Here's how the part is built. I have some questions about the finished solid (model axes, mm). Coordinates: 2 decimals unless noted, no trailing zeros. Loops run counter-clockwise (first coordinate to the right, second up) from the corner with the lowest first, then second, coordinate; pieces in that order, holes last. Notation, with made-up numbers: M 88,27 L 109,27 A31 ccw 109,62 Z; hole C 54,23.25 d5. An arc over 180 degrees is marked long. Use CSV: the item, a comma, the result in double quotes. Start each with the question number.
Q1. If we section it at D-D (y = 5): State how many separate pieces and enclosed holes the cut face has, and give its area (3 significant figures).
Q2. Please list where these lines run through material, in increasing order: probe 1 along X at (y, z) = (5, -1.55); probe 2 along Y at (x, z) = (-45, -2.2); probe 3 along Y at (x, z) = (-65, 0). Write a range as [from, to].
Q3. If we mould it in two halves opening along Y, with no side actions, what happens to faces 1 (the flat face through (-1, 0, 5)), 2 (the conical face through (-22.059, 3.125, 2.188)), 3 (the flat face through (1, 25, 0)), 4 (the cylindrical face through (-22.07, 3.48, -1.55))? For each: +Y half, -Y half, draft (parallel to the pull), parting line (faces both ways), or undercut.
Q4. For pin 1 Ø6 at (x, y) = (-25, 5) entering from -Z, with a flat end and sliding along its axis, tell me the tip position at first contact or that it passes through.
Q5. If we section it at B-B (z = -2): Please give me the cut outline in (x, y).
Q6. If we section it at A-A (x = -25): Please give me the cut outline in (y, z).
Q7. If we section it at C-C (x = -45): Please give me the cut outline in (y, z), and give its area (3 significant figures).
Autodesk Inventor part; units mm, degrees
ref_plane "YZ Plane" through (0, 0, 0) normal (1, 0, 0) x (0, 1, 0)
ref_plane "XZ Plane" through (0, 0, 0) normal (0, 1, 0) x (-1, 0, 0)
ref_plane "XY Plane" through (0, 0, 0) normal (0, 0, 1) x (1, 0, 0)
sketch "Sketch2" plane through (0, 0, 0) normal (0, 0, 1) x (1, 0, 0)
  line L0 (-75, -25) -> (75, -25)
  line L1 (75, -25) -> (75, 25)
  line L2 (75, 25) -> (-75, 25)
  line L3 (-75, 25) -> (-75, -25)
  line L4 (-75, -25) -> (75, 25) construction
  line L5 (75, -25) -> (-75, 25) construction
  point P0 (0, 0)
  dimension "d1" = 150
  dimension "d2" = 50
extrude "Extrusion1" add sketch "Sketch2" along normal mid plane 10
sketch "Sketch3" plane through (0, 0, 5) normal (0, 0, 1) x (1, 0, 0)
  line L0 (-75, 25) -> (-75, -25)
  line L1 (75, 25) -> (-75, 25)
  point P0 (0, 0)
  point P1 (-65, 0)
  dimension "d40" = 10
  dimension "d43" = 25
hole "Hole1" at (-65, 0, 5) direction (0, 0, -1) diameter 6.6 depth 14.2 tip angle 118 countersink diameter 12.6 countersink angle 90
sketch "Sketch4" plane through (0, 0, 5) normal (0, 0, 1) x (1, 0, 0)
  line L0 (-75, 25) -> (-75, -25)
  line L1 (75, 25) -> (-75, 25)
  point P0 (0, 0)
  point P1 (-45, 5)
  dimension "d41" = 30
  dimension "d42" = 20
hole "Hole2" at (-45, 5, 5) direction (0, 0, -1) diameter 9 depth 14.2 tip angle 118 countersink diameter 17.3 countersink angle 90
sketch "Sketch5" plane through (0, 0, 5) normal (0, 0, 1) x (1, 0, 0)
  line L0 (-75, 25) -> (-75, -25)
  line L1 (75, 25) -> (-75, 25)
  point P0 (0, 0)
  point P1 (-25, 5)
  dimension "d44" = 50
  dimension "d45" = 20
hole "Hole3" at (-25, 5, 5) direction (0, 0, -1) diameter 6.6 depth 14.2 tip angle 118 countersink diameter 12.6 countersink angle 90
properties part number "홀간 거리 확인 파트-10_CPY" material "SS400"
Results below:
1,separate pieces,"3"
1,enclosed holes,"0"
1,area,"1,310 mm^2"
2,probe 1,"[-75, -49.5], [-40.5, -28.3], [-21.7, 75]"
2,probe 2,"[-25, 0.5], [9.5, 25]"
2,probe 3,"[-25, -3.3], [3.3, 25]"
3,face 1,"draft"
3,face 2,"undercut"
3,face 3,"+Y half"
3,face 4,"undercut"
4,pin 1,"through"
5,outline,"M -75,-25 L 75,-25 L 75,25 L -75,25 Z; hole C -65,0 d6.6; hole C -45,5 d9; hole C -25,5 d6.6"
6,outline,"M -25,-5 L 1.7,-5 L 1.7,2 L -1.3,5 L -25,5 Z; M 8.3,-5 L 25,-5 L 25,5 L 11.3,5 L 8.3,2 Z"
7,outline,"M -25,-5 L 0.5,-5 L 0.5,0.85 L -3.65,5 L -25,5 Z; M 9.5,-5 L 25,-5 L 25,5 L 13.65,5 L 9.5,0.85 Z"
7,area,"393 mm^2"
